```python
from build123d import *

# Parameters (mm, degrees)
SKETCH1_R           = 20
SKETCH1_R_2         = 1
BOSS_EXTRUDE1_DEPTH = 2
SKETCH2_R           = 20
SKETCH2_R_2         = 1
SKETCH2_R_3         = 2.3
BOSS_EXTRUDE3_DEPTH = 8
BOSS_EXTRUDE4_DEPTH = 5
SKETCH4_R           = 2.3
SKETCH4_R_2         = 1.05
BOSS_EXTRUDE5_DEPTH = 2
SKETCH5_R           = 0.740059644
CUT_EXTRUDE1_DEPTH  = 6


with BuildPart() as part:
    # Sketch1 → Boss-Extrude1 (new body)
    with BuildSketch(Plane(origin=(0, 0, 0), x_dir=(1, 0, 0), z_dir=(0, 1, 0))):
        with Locations((-25.651058935, -9.088114724)):
            Circle(SKETCH1_R)
        with Locations((-17.747716132, 3.008978834)):
            Circle(SKETCH1_R_2, mode=Mode.SUBTRACT)
        with Locations((-33.554401738, -21.185208281)):
            Circle(SKETCH1_R_2, mode=Mode.SUBTRACT)
        with BuildLine():
            ThreePointArc((-20.532647943, -4.727567864), (-21.084075378, -2.097752703), (-23.713890539, -2.649180137))
            Line((-23.713890539, -2.649180137), (-25.439308031, -5.290155905))
            Line((-25.439308031, -5.290155905), (-38.480446345, 1.673359092))
            ThreePointArc((-38.480446345, 1.673359092), (-41.09682891, 1.003004634), (-40.659707143, -1.662282853))
            Line((-40.659707143, -1.662282853), (-29.044052435, -10.807685815))
            Line((-29.044052435, -10.807685815), (-30.769469927, -13.448661583))
            ThreePointArc((-30.769469927, -13.448661583), (-30.218042492, -16.078476745), (-27.588227331, -15.52704931))
            Line((-27.588227331, -15.52704931), (-25.63545633, -12.538079442))
            Line((-25.63545633, -12.538079442), (-25.251093904, -12.514851944))
            Line((-25.251093904, -12.514851944), (-14.889738345, -18.504207673))
            ThreePointArc((-14.889738345, -18.504207673), (-12.21449481, -17.866568148), (-12.705220614, -15.16051931))
            Line((-12.705220614, -15.16051931), (-22.35228997, -8.077855691))
            Line((-22.35228997, -8.077855691), (-22.485418943, -7.716537732))
            Line((-22.485418943, -7.716537732), (-20.532647943, -4.727567864))
        make_face(mode=Mode.SUBTRACT)
    extrude(amount=BOSS_EXTRUDE1_DEPTH)

    # Sketch2 → Boss-Extrude3 (add)
    with BuildSketch(Plane.XZ):
        with Locations((-25.651058935, 9.088114724)):
            Circle(SKETCH2_R)
        with Locations((-17.747716132, -3.008978834)):
            Circle(SKETCH2_R_2, mode=Mode.SUBTRACT)
        with Locations((-33.554401738, 21.185208281)):
            Circle(SKETCH2_R_2, mode=Mode.SUBTRACT)
        with Locations((-25.651058935, 9.088114724)):
            Circle(SKETCH2_R_3, mode=Mode.SUBTRACT)
    extrude(amount=BOSS_EXTRUDE3_DEPTH)

    # Sketch3 → Boss-Extrude4 (add)
    with BuildSketch(Plane.XZ.offset(8)):
        with BuildLine():
            Line((-23.725569995, 10.346086242), (-26.460290688, 14.531931764))
            Line((-26.460290688, 14.531931764), (-12.174069633, 23.865487946))
            ThreePointArc((-12.174069633, 23.865487946), (-8.907676848, 20.026997496), (-6.704628247, 15.493796903))
            Line((-6.704628247, 15.493796903), (-20.990849302, 6.160240721))
            Line((-20.990849302, 6.160240721), (-23.725569995, 10.346086242))
        make_face()
        with BuildLine():
            Line((-27.576547875, 7.830143205), (-24.841827182, 3.644297683))
            Line((-24.841827182, 3.644297683), (-39.128048237, -5.689258499))
            ThreePointArc((-39.128048237, -5.689258499), (-42.394441021, -1.850768048), (-44.597489623, 2.682432545))
            Line((-44.597489623, 2.682432545), (-30.311268568, 12.015988727))
            Line((-30.311268568, 12.015988727), (-27.576547875, 7.830143205))
        make_face()
    extrude(amount=BOSS_EXTRUDE4_DEPTH)

    # Sketch4 → Boss-Extrude5 (add)
    with BuildSketch(Plane(origin=(0, 0, 0), x_dir=(1, 0, 0), z_dir=(0, 1, 0))):
        with Locations((-25.651058935, -9.088114724)):
            Circle(SKETCH4_R)
        with Locations((-25.651058935, -9.088114724)):
            Circle(SKETCH4_R_2, mode=Mode.SUBTRACT)
    extrude(amount=-BOSS_EXTRUDE5_DEPTH)

    # Sketch5 → Cut-Extrude1 (cut)
    with BuildSketch(Plane(origin=(0, 2, 0), x_dir=(1, 0, 0), z_dir=(0, 1, 0))):
        with Locations((-20.12753999, 54.77317824)):
            Circle(SKETCH5_R)
    extrude(amount=-CUT_EXTRUDE1_DEPTH, mode=Mode.SUBTRACT)


solid = part.part
```
Here's how the part is built. I have some questions about the finished solid (model axes, mm). A direction names the side the tool comes from. Give positions to 0.01 mm unless a question says otherwise; leave off trailing zeros. Loops run counter-clockwise (first coordinate to the right, second up) from the corner with the lowest first, then second, coordinate; pieces in that order, holes last. Notation, with made-up numbers: M 32.25,-38 L 86.25,-38 A8 cw 86.25,-23 Z; hole C 74.5,34 d9. An arc over 180 degrees is marked long. Use one line per item in the form item = value. Start each with the question number.
Q1. Which directions (+Z, -Z, +X, -X, +Y, -Y) give clear straight access to the entire face, cutting with the end or side of a thin tool? Please do faces 5 (the flat face through (-27, -2, 9)), 6 (the flat face through (-25.9, 2, 13.3)), 7 (the flat face through (-24.565, 0.986, 3.951)).
Q2. If we section it at B-B (y = 0.5): Write out the boundary of the cut face in (x, z).
Q3. Will these pins go through, and if not, where does the flat tip stop? pin 1 Ø8 at (y, z) = (-6.5, 19.5) entering from -X; pin 2 Ø1.8 at (x, z) = (-17.75, -3.01) entering from -Y; pin 3 Ø6 at (x, y) = (-39, -2) entering from -Z; pin 4 Ø8 at (x, z) = (-18, -1) entering from -Y.
Q4. If we section it at A-A (y = -10.75): Write out the boundary of the cut face in (x, z).
Q5. If we section it at C-C (x = -9.5): Write out the boundary of the cut face in (y, z).
Q6. If we section it at D-D (z = 26): Write out the boundary of the cut face in (x, y).
Q7. I need wall thicknesses on line 1 along Z through (x, y) = (-30.5, 1.5); line 2 along Y through (x, z) = (-16, -3); line 3 along Z through (x, y) = (-24.5, -6.5). Which ranges of each line are inside material? Lowest first, please.
Q8. Thinking about a two-plate mould opening in Z: for faces 1 (the flat face through (-19.42, -10.46, 19.13)), 2 (the flat face through (-13.75, -10.46, 10.89)), 3 (the flat face through (-35, -13, 3)), 4 (the flat face through (-21.52, 0.99, 6.24)), which applies, +Z half, -Z half, draft (parallel to the pull), parting line (faces both ways), or undercut?
Taken from the geometry:
q1.face_5 = -Y
q1.face_6 = +Z, -Z, +X, -X, +Y
q1.face_7 = +Y
q2.outline = C -25.65,9.09 d40; hole M -40.66,1.66 A2 ccw -38.48,-1.67 L -25.44,5.29 L -23.71,2.65 A1.9 ccw -20.53,4.73 L -22.49,7.72 L -22.35,8.08 L -12.71,15.16 A2 ccw -14.89,18.5 L -25.25,12.51 L -25.64,12.54 L -27.59,15.53 A1.9 ccw -30.77,13.45 L -29.04,10.81 Z; hole C -33.55,21.19 d2; hole C -17.75,-3.01 d2
q3.pin_1 = -44.6
q3.pin_2 = through
q3.pin_3 = -8.03
q3.pin_4 = -8
q4.outline = M -44.6,2.68 A20 ccw -39.13,-5.69 L -24.84,3.64 L -30.31,12.02 Z; M -26.46,14.53 L -20.99,6.16 L -6.7,15.49 A20 ccw -12.17,23.87 Z
q5.outline = M -13,13.67 L -8,13.67 L -8,-2.71 L 2,-2.71 L 2,20.88 L -13,20.88 Z
q6.outline = M -36.33,-8 L -14.97,-8 L -14.97,2 L -36.33,2 Z
q7.line_1 = -10.32 to 2.59, 9.66 to 13.04, 15.85 to 28.49
q7.line_2 = -8 to 2
q7.line_3 = -10.88 to 7.1, 11.08 to 29.05
q8.face_1 = +Z half
q8.face_2 = -Z half
q8.face_3 = draft
q8.face_4 = undercut
